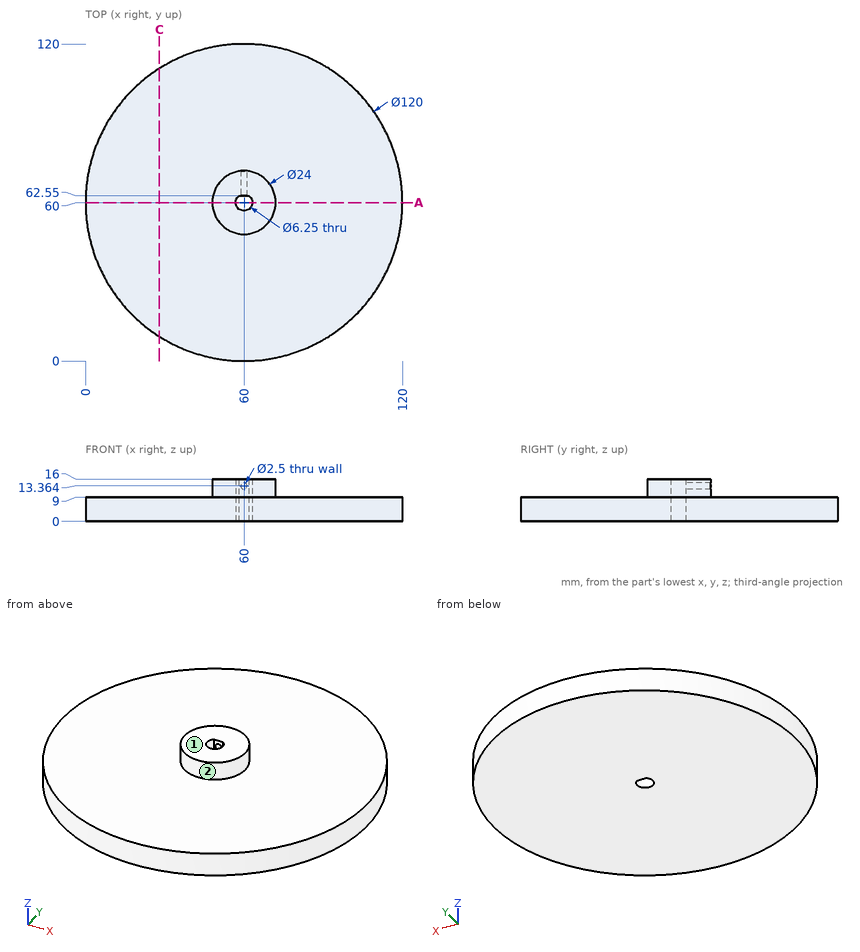
Part print with two shaded views. Sizes in mm from the minimum x, y, z corner. A direction names the side the tool comes from. Round coordinates to 2 decimals unless told otherwise and drop trailing zeros. Loops run counter-clockwise (first coordinate to the right, second up) from the corner with the lowest first, then second, coordinate; pieces in that order, holes last. Notation, with made-up numbers: M 84,-7.75 L 98,-7.75 A29 cw 98,17.25 Z; hole C 76,74 d1. An arc over 180 degrees is marked long. Return JSON: item names as keys, results as strings. Group by question number.
(1) Tool access for the marked faces 1 and 2: list every direction of +Z, -Z, +X, -X, +Y, -Y with a clear straight run to the whole face (end or side of a thin tool).
(2) Saw through at A-A, the plane y = 60. List the corners of the cut face in (x, z) (3 decimals).
(3) Saw through at C-C, the plane x = 28. List the corners of the cut face in (y, z).
(4) Drop flat-ended pins along their axis: P1, Ø1, axis at x = 19.5, z = 5.5, coming from the -Y side; P2, Ø1.5, axis at x = 52.5, z = 5, coming from the +Y side; P3, Ø4, axis at x = 60, z = 13.36, coming from the +Y side. Give the stop position or say it passes through.
(5) Wall check: probe 1 along Y at (x, z) = (60, 6) (3 decimals); probe 2 along Z at (x, y) = (60, 67); probe 3 along Y at (x, z) = (60, 10.5) (3 decimals). Give the ranges that are in metal, low to high. Write a range as [from, to].
Answer list:
{
 "1": {"face 1": "+Z, +X, -X, +Y, -Y", "face 2": "+Z"},
 "2": {"outline": "M 0,0 L 56.875,0 L 56.875,16 L 48,16 L 48,9 L 0,9 Z; M 63.125,0 L 120,0 L 120,9 L 72,9 L 72,16 L 63.125,16 Z"},
 "3": {"outline": "M 9.25,0 L 110.75,0 L 110.75,9 L 9.25,9 Z"},
 "4": {"P1": "y = 15.28", "P2": "y = 119.62", "P3": "y = 72"},
 "5": {"probe 1": "[0, 56.875], [62.55, 120]", "probe 2": "[0, 12.11], [14.61, 16]", "probe 3": "[48, 56.875], [62.55, 72]"}
}
